For this review, take the finished solid that the model builds, in its own axes (mm). A direction names the side the tool comes from. Round coordinates to 2 decimals unless told otherwise and drop trailing zeros. Write each loop counter-clockwise with the first axis right and the second up, starting at its lowest first coordinate (ties: lowest second). Pieces come first, ordered by that corner, then holes.
from build123d import *

# Parameters (mm, degrees)
BOSS_EXTRUDE1_DEPTH = 100
CUT_EXTRUDE1_REACH  = 167.428
SKETCH2_R           = 40
FILLET2_R           = 5


with BuildPart() as part:
    # Sketch1 → Boss-Extrude1 (new body)
    with BuildSketch(Plane(origin=(0, 0, 0), x_dir=(1, 0, 0), z_dir=(0, 1, 0))):
        Polygon((50.3, -110), (50.3, -10.392304845), (68.3, 0), (68.3, 112.701705922), (50.3, 112.701705922), (50.3, 12.701705922), (28.3, 0), (0, 0), (0, -110), align=None)
    extrude(amount=BOSS_EXTRUDE1_DEPTH)

    # Sketch2 → Cut-Extrude1 (cut, up to next)
    with BuildSketch(Plane(origin=(68.3, 0, 0), x_dir=(0, 0, -1), z_dir=(1, 0, 0)), mode=Mode.PRIVATE) as cut_extrude1_sk1:
        with Locations((56.350852961, 50)):
            Circle(SKETCH2_R)
    cut_extrude1_tool1 = extrude(cut_extrude1_sk1.sketch, amount=-CUT_EXTRUDE1_REACH, mode=Mode.PRIVATE) & part.part
    add(cut_extrude1_tool1.solids().sort_by_distance((68.3, 50, -56.350853))[0], mode=Mode.SUBTRACT)

    # Fillet2
    fillet2_edges = [part.edges().sort_by_distance(p)[0] for p in [
        (50.3, 0, 60.196152423),
        (50.3, 100, 60.196152423),
        (59.3, 0, 5.196152423),
        (59.3, 100, 5.196152423),
        (68.3, 0, -56.350852961),
        (68.3, 50, -112.701705922),
        (68.3, 100, -56.350852961),
        (68.3, 50, 0),
        (50.3, 50, 10.392304845),
        (59.3, 0, -112.701705922),
        (59.3, 100, -112.701705922),
    ]]
    fillet(fillet2_edges, radius=FILLET2_R)


solid = part.part
(1) We need section B-B, the plane z = -61. Give the boundary of the cut face in (x, y).
Geometry check:
outline: (50.3, 0) - (63.3, 0) arc R5 ccw to (68.3, 5) - (68.3, 10.27) - (50.3, 10.27) - close; (50.3, 89.73) - (68.3, 89.73) - (68.3, 95) arc R5 ccw to (63.3, 100) - (50.3, 100) - close
(2) We need section D-D, the plane y = 31. Give the boundary of the cut face in (x, z).
Geometry check:
outline: (0, 0) - (28.3, 0) - (50.3, -12.7) - (50.3, -21.15) - (68.3, -21.15) - (68.3, -2.89) arc R5 ccw to (65.8, 1.44) - (52.8, 8.95) arc R5 cw to (50.3, 13.28) - (50.3, 110) - (0, 110) - close; (50.3, -112.7) - (63.3, -112.7) arc R5 ccw to (68.3, -107.7) - (68.3, -91.55) - (50.3, -91.55) - close
(3) For pin 1 Ø12 at (y, z) = (10, -38.5) entering from -X; pin 2 Ø22.5 at (x, y) = (11, 41) entering from -Z; pin 3 Ø8 at (x, z) = (55.5, 73.5) entering from -Y, all flat-tipped, find the tip position at first contact; note any pin that passes through.
Geometry check:
pin 1: stops at x = 50.3
pin 2: stops at z = 0
pin 3: passes through
(4) For line 1 along X through (y, z) = (13, 81); line 2 along Z through (x, y) = (14, 80); line 3 along Z through (x, y) = (52.5, 67.5), list the stretches that pass through material, from the lowest coordinate up.
Geometry check:
line 1: x = 0 to 50.3
line 2: z = 0 to 110
line 3: z = -112.7 to -92.32, -20.38 to 9.14
(5) Mouldability with a two-part tool opening along Y and no side actions: class faces 1 (the face through (56.71, 1.43, -111.2)), 2 (the face through (68.3, 29, -20)), 3 (the face through (59.426, 14.513, -74.808)) as pulls with the +Y half, pulls with the -Y half, needs draft (parallel to the pull), parting line crosses it, or undercut.
Geometry check:
face 1: pulls with the -Y half
face 2: needs draft
face 3: undercut
(6) We need section A-A, the plane y = 50. Give the boundary of the cut face in (x, z), and give its area (3 significant figures).
Geometry check:
outline: (0, 0) - (28.3, 0) - (50.3, -12.7) - (50.3, -16.35) - (68.3, -16.35) - (68.3, -2.89) arc R5 ccw to (65.8, 1.44) - (52.8, 8.95) arc R5 cw to (50.3, 13.28) - (50.3, 110) - (0, 110) - close; (50.3, -112.7) - (63.3, -112.7) arc R5 ccw to (68.3, -107.7) - (68.3, -96.35) - (50.3, -96.35) - close
area: 6,350 mm2
(7) For faces 4 (the face through (50.3, 49, 62)), 5 (the face through (48.87, 98.5, 60.96)), 6 (the face through (50.3, 49, -97)), 7 (the face through (57, 49, -112.702)), 8 (the face through (48.87, 1.5, 60.96)), list the 3-axis set-ups (+Z, -Z, +X, -X, +Y, -Y) from which the entire face can be reached by the end or side of a thin tool; tool diameter is ignored.
Geometry check:
face 4: +Z, +X, +Y, -Y
face 5: +Z, +X, +Y
face 6: -Z, -X, +Y, -Y
face 7: -Z, +X, -X, +Y, -Y
face 8: +Z, +X, -Y
(8) We need section C-C, the plane z = 34.5. Give the boundary of the cut face in (x, y).
Geometry check:
outline: (0, 0) - (45.3, 0) arc R5 ccw to (50.3, 5) - (50.3, 95) arc R5 ccw to (45.3, 100) - (0, 100) - close
